CAD build for the part. Positions are in the model's coordinates, mm. Coordinates: 2 decimals unless noted, no trailing zeros. Order: outer loops, then holes, each group sorted by start corner. A loop starts at its lowest first (then second) coordinate and runs counter-clockwise, first axis right, second up. Notation, with made-up numbers: M 16,33 L 29,33 A20 ccw 29,44 Z; hole C 67,10 d2. An arc over 180 degrees is marked long. One line per item, written item: value.
from build123d import *

# Parameters (mm, degrees)
SKETCH1_W                      = 250
SKETCH1_H                      = 66.3
BOSS_EXTRUDE1_DEPTH            = 4
F_5_0MM_DOWEL_HOLE2_AT_2_COUNT = 2
F_5_0MM_DOWEL_HOLE2_AT_2_PITCH = 9
LPATTERN2_COUNT                = 2
LPATTERN2_PITCH                = 65


with BuildPart() as part:
    # Sketch1 → Boss-Extrude1 (new body)
    with BuildSketch(Plane(origin=(0, 0, 0), x_dir=(1, 0, 0), z_dir=(0, 1, 0))):
        Rectangle(SKETCH1_W, SKETCH1_H)
    extrude(amount=BOSS_EXTRUDE1_DEPTH)

    # Sketch5 → Ø3.0mm Dowel Hole1 (revolve, cut)
    with BuildSketch(Plane(origin=(-114.5, 4, 0), x_dir=(0, 0, 1), z_dir=(1, 0, 0))):
        Polygon((0, 0), (0, 100.901290929), (1.5, 100), (1.5, 0), align=None)
    f_3_0mm_dowel_hole1 = revolve(axis=Axis((-114.5, 10.35, 0), (0, -1, 0)), mode=Mode.SUBTRACT)

    # Sketch7 → Ø5.0mm Dowel Hole2 (revolve, cut)
    with BuildSketch(Plane(origin=(-95, 4, -22.15), x_dir=(0, 0, 1), z_dir=(1, 0, 0))):
        Polygon((0, 0), (0, 51.502151548), (2.5, 50), (2.5, 0), align=None)
    f_5_0mm_dowel_hole2 = revolve(axis=Axis((-95, 10.35, -22.15), (0, -1, 0)), mode=Mode.SUBTRACT)

    # Ø5.0mm Dowel Hole2 at 2: Ø5.0mm Dowel Hole2 ×2
    with Locations(*[(0, 0, i * F_5_0MM_DOWEL_HOLE2_AT_2_PITCH) for i in range(1, F_5_0MM_DOWEL_HOLE2_AT_2_COUNT)]):
        add(f_5_0mm_dowel_hole2, mode=Mode.SUBTRACT)

    # LPattern2: Ø5.0mm Dowel Hole2 ×2
    with Locations(*[(i * LPATTERN2_PITCH, 0, 0) for i in range(1, LPATTERN2_COUNT)]):
        add(f_5_0mm_dowel_hole2, mode=Mode.SUBTRACT)

    # LPattern2 copy 1 sketch → LPattern2 copy 1 (revolve, cut)
    with BuildSketch(Plane(origin=(-30, 4, -13.15), x_dir=(0, 0, 1), z_dir=(1, 0, 0))):
        Polygon((0, 0), (0, 51.502151548), (2.5, 50), (2.5, 0), align=None)
    revolve(axis=Axis((-30, 10.35, -13.15), (0, -1, 0)), mode=Mode.SUBTRACT)

    # Mirror3: Ø3.0mm Dowel Hole1, Ø5.0mm Dowel Hole2 across plane
    add(f_3_0mm_dowel_hole1.mirror(Plane(origin=(0, 0, 0), x_dir=(0, 0, 1), z_dir=(1, 0, 0))), mode=Mode.SUBTRACT)
    add(f_5_0mm_dowel_hole2.mirror(Plane(origin=(0, 0, 0), x_dir=(0, 0, 1), z_dir=(1, 0, 0))), mode=Mode.SUBTRACT)

    # Mirror3 copy 1 sketch → Mirror3 copy 1 (revolve, cut)
    with BuildSketch(Plane(origin=(95, 4, -13.15), x_dir=(0, 0, 1), z_dir=(-1, 0, 0))):
        Polygon((0, 0), (0, -51.502151548), (2.5, -50), (2.5, 0), align=None)
    revolve(axis=Axis((95, 10.35, -13.15), (0, 1, 0)), mode=Mode.SUBTRACT)

    # Mirror3 copy 2 sketch → Mirror3 copy 2 (revolve, cut)
    with BuildSketch(Plane(origin=(30, 4, -22.15), x_dir=(0, 0, 1), z_dir=(-1, 0, 0))):
        Polygon((0, 0), (0, -51.502151548), (2.5, -50), (2.5, 0), align=None)
    revolve(axis=Axis((30, 10.35, -22.15), (0, 1, 0)), mode=Mode.SUBTRACT)

    # Mirror3 copy 3 sketch → Mirror3 copy 3 (revolve, cut)
    with BuildSketch(Plane(origin=(30, 4, -13.15), x_dir=(0, 0, 1), z_dir=(-1, 0, 0))):
        Polygon((0, 0), (0, -51.502151548), (2.5, -50), (2.5, 0), align=None)
    revolve(axis=Axis((30, 10.35, -13.15), (0, 1, 0)), mode=Mode.SUBTRACT)

    # Mirror4: Ø5.0mm Dowel Hole2 across plane
    add(f_5_0mm_dowel_hole2.mirror(Plane.XY), mode=Mode.SUBTRACT)

    # Mirror4 copy 1 sketch → Mirror4 copy 1 (revolve, cut)
    with BuildSketch(Plane(origin=(-95, 4, 13.15), x_dir=(0, 0, -1), z_dir=(1, 0, 0))):
        Polygon((0, 0), (0, -51.502151548), (2.5, -50), (2.5, 0), align=None)
    revolve(axis=Axis((-95, 10.35, 13.15), (0, 1, 0)), mode=Mode.SUBTRACT)

    # Mirror4 copy 2 sketch → Mirror4 copy 2 (revolve, cut)
    with BuildSketch(Plane(origin=(-30, 4, 22.15), x_dir=(0, 0, -1), z_dir=(1, 0, 0))):
        Polygon((0, 0), (0, -51.502151548), (2.5, -50), (2.5, 0), align=None)
    revolve(axis=Axis((-30, 10.35, 22.15), (0, 1, 0)), mode=Mode.SUBTRACT)

    # Mirror4 copy 3 sketch → Mirror4 copy 3 (revolve, cut)
    with BuildSketch(Plane(origin=(-30, 4, 13.15), x_dir=(0, 0, -1), z_dir=(1, 0, 0))):
        Polygon((0, 0), (0, -51.502151548), (2.5, -50), (2.5, 0), align=None)
    revolve(axis=Axis((-30, 10.35, 13.15), (0, 1, 0)), mode=Mode.SUBTRACT)

    # Mirror4 copy 4 sketch → Mirror4 copy 4 (revolve, cut)
    with BuildSketch(Plane(origin=(114.5, 4, 0), x_dir=(0, 0, -1), z_dir=(-1, 0, 0))):
        Polygon((0, 0), (0, 100.901290929), (1.5, 100), (1.5, 0), align=None)
    revolve(axis=Axis((114.5, 10.35, 0), (0, -1, 0)), mode=Mode.SUBTRACT)

    # Mirror4 copy 5 sketch → Mirror4 copy 5 (revolve, cut)
    with BuildSketch(Plane(origin=(95, 4, 22.15), x_dir=(0, 0, -1), z_dir=(-1, 0, 0))):
        Polygon((0, 0), (0, 51.502151548), (2.5, 50), (2.5, 0), align=None)
    revolve(axis=Axis((95, 10.35, 22.15), (0, -1, 0)), mode=Mode.SUBTRACT)

    # Mirror4 copy 6 sketch → Mirror4 copy 6 (revolve, cut)
    with BuildSketch(Plane(origin=(95, 4, 13.15), x_dir=(0, 0, -1), z_dir=(-1, 0, 0))):
        Polygon((0, 0), (0, 51.502151548), (2.5, 50), (2.5, 0), align=None)
    revolve(axis=Axis((95, 10.35, 13.15), (0, -1, 0)), mode=Mode.SUBTRACT)

    # Mirror4 copy 7 sketch → Mirror4 copy 7 (revolve, cut)
    with BuildSketch(Plane(origin=(30, 4, 22.15), x_dir=(0, 0, -1), z_dir=(-1, 0, 0))):
        Polygon((0, 0), (0, 51.502151548), (2.5, 50), (2.5, 0), align=None)
    revolve(axis=Axis((30, 10.35, 22.15), (0, -1, 0)), mode=Mode.SUBTRACT)

    # Mirror4 copy 8 sketch → Mirror4 copy 8 (revolve, cut)
    with BuildSketch(Plane(origin=(30, 4, 13.15), x_dir=(0, 0, -1), z_dir=(-1, 0, 0))):
        Polygon((0, 0), (0, 51.502151548), (2.5, 50), (2.5, 0), align=None)
    revolve(axis=Axis((30, 10.35, 13.15), (0, -1, 0)), mode=Mode.SUBTRACT)

    # Mirror4 copy 9 sketch → Mirror4 copy 9 (revolve, cut)
    with BuildSketch(Plane(origin=(-114.5, 4, 0), x_dir=(0, 0, -1), z_dir=(1, 0, 0))):
        Polygon((0, 0), (0, -100.901290929), (1.5, -100), (1.5, 0), align=None)
    revolve(axis=Axis((-114.5, 10.35, 0), (0, 1, 0)), mode=Mode.SUBTRACT)


solid = part.part
Q1. Mould opens along X. For faces 1 (the face through (-97.48, 2.03, -22.48)), 2 (the face through (125, 2, 0)), 3 (the face through (-2, 4, 0)), 4 (the face through (-31.69, 2.03, -14.99)) say: released by +X, released by -X, zero draft, split by the parting line, or undercut.
Recorded:
face 1: undercut
face 2: released by +X
face 3: zero draft
face 4: undercut
Q2. Pin check, flat tip, straight feed: pin 1 Ø2.5 at (x, z) = (114.5, 0) entering from +Y. Stop position of the tip, or through.
Recorded:
pin 1: passes through
Q3. Slice it at C-C (x = 95). List the corners of the cut face in (y, z).
Recorded:
outline: M 0,-33.15 L 4,-33.15 L 4,-24.65 L 0,-24.65 Z; M 0,-19.65 L 4,-19.65 L 4,-15.65 L 0,-15.65 Z; M 0,-10.65 L 4,-10.65 L 4,10.65 L 0,10.65 Z; M 0,15.65 L 4,15.65 L 4,19.65 L 0,19.65 Z; M 0,24.65 L 4,24.65 L 4,33.15 L 0,33.15 Z
Q4. Slice it at A-A (z = -13.15). List the corners of the cut face in (x, y), plus the area to 3 significant figures.
Recorded:
outline: M -125,0 L -97.5,0 L -97.5,4 L -125,4 Z; M -92.5,0 L -32.5,0 L -32.5,4 L -92.5,4 Z; M -27.5,0 L 27.5,0 L 27.5,4 L -27.5,4 Z; M 32.5,0 L 92.5,0 L 92.5,4 L 32.5,4 Z; M 97.5,0 L 125,0 L 125,4 L 97.5,4 Z
area: 920 mm^2
Q5. Drill centre lines: line 1 along Z through (x, y) = (-30, 2.15); line 2 along Z through (x, y) = (-114.5, 2.15); line 3 along X through (y, z) = (1.8, -23.5). Where is each one in solid material? Low to high.
Recorded:
line 1: z = -33.15 to -24.65, -19.65 to -15.65, -10.65 to 10.65, 15.65 to 19.65, 24.65 to 33.15
line 2: z = -33.15 to -1.5, 1.5 to 33.15
line 3: x = -125 to -97.1, -92.9 to -32.1, -27.9 to 27.9, 32.1 to 92.9, 97.1 to 125
Q6. Slice it at B-B (y = 1.8). Give the number of separate pieces and of enclosed holes in the cut face, plus the area to 3 significant figures.
Recorded:
separate pieces: 1
enclosed holes: 18
area: 16,200 mm^2
